Read the model definition and answer for the solid it produces. Units are mm, in the model's axes. A direction names the side the tool comes from. Give positions to 0.01 mm unless a question says otherwise; leave off trailing zeros. Loops run counter-clockwise (first coordinate to the right, second up) from the corner with the lowest first, then second, coordinate; pieces in that order, holes last. Notation, with made-up numbers: (-17, -31) - (39, -31) arc R18 cw to (39, -14) - close; hole circle Ø11 at (48.25, 23). An arc over 180 degrees is marked (long way). Write each question's results on one line, items separated by ' | '. Start each with the question number.
Q1. Find the intervals of material crossed by line 1 (X direction, y = 0, z = -17); line 2 (X direction, y = -11, z = -17); line 3 (Y direction, x = -15.5, z = 18), in increasing order. Write a range as from..to.
Q2. For faces 4 (the flat face through (-11.737, -10.552, -0.338)), 5 (the flat face through (0.838, 16, 0)), 6 (the flat face through (-0.838, -16, 0)), 7 (the flat face through (11.737, 10.552, -0.338)), determine the directions among +Z, -Z, +X, -X, +Y, -Y from which every point of the face is accessible in a straight line to the end or side of a thin tool.
Q3. The part is cut by section D-D, the plane y = -17. Write down the section's boundary in (x, z).
Q4. Given pin 1 (3 mm diameter, centred on x = -13, y = 7, fed in from +Z); pin 2 (12 mm diameter, centred on y = 3.5, z = -5.5, fed in from -X); pin 3 (5.5 mm diameter, centred on x = 16.5, z = 0, fed in from +Y); pin 4 (4 mm diameter, centred on x = -11.5, z = -8, fed in from -Y), each flat-ended and moving along its own axis, determine where each tip first touches the part or whether it passes through.
Q5. The part is cut by section A-A, the plane y = -9. Write down the section's boundary in (x, z).
Q6. The part is cut by section C-C, the plane y = 3. Write down the section's boundary in (x, z), plus the area to 3 significant figures.
Q7. Determine the mould class of faces 1 (the flat face through (-0.838, 16, 0)), 2 (the flat face through (-16, -0.838, 0)), 3 (the flat face through (0, -21.555, 0)) for opening direction Y: +Y half, -Y half, draft (parallel to the pull), parting line (faces both ways), or undercut.
Q8. The part is cut by section B-B, the plane x = 5. Write down the section's boundary in (y, z), plus the area to 3 significant figures.
Autodesk Inventor part; units mm, degrees
ref_plane "YZ Plane" through (0, 0, 0) normal (1, 0, 0) x (0, 1, 0)
ref_plane "XZ Plane" through (0, 0, 0) normal (0, 1, 0) x (-1, 0, 0)
ref_plane "XY Plane" through (0, 0, 0) normal (0, 0, 1) x (1, 0, 0)
sketch "Sketch1" plane through (0, 0, 0) normal (0, 0, 1) x (1, 0, 0)
  circle A0 centre (0, 0) radius 10.16
  circle A1 centre (0, 0) radius 8.5725
  line L0 (0.8382, 10.1254) -> (0.8382, 21.5554)
  line L1 (0.8382, 21.5554) -> (-0.8382, 21.5554)
  line L2 (-0.8382, 21.5554) -> (-0.8382, 10.1254)
  line L3 (-15.8346, 14.6492) -> (-7.7524, 6.567)
  line L4 (-14.6492, 15.8346) -> (-15.8346, 14.6492)
  line L5 (-6.567, 7.7524) -> (-14.6492, 15.8346)
  line L6 (-21.5554, -0.8382) -> (-10.1254, -0.8382)
  line L7 (-21.5554, 0.8382) -> (-21.5554, -0.8382)
  line L8 (-10.1254, 0.8382) -> (-21.5554, 0.8382)
  line L9 (-14.6492, -15.8346) -> (-6.567, -7.7524)
  line L10 (-15.8346, -14.6492) -> (-14.6492, -15.8346)
  line L11 (-7.7524, -6.567) -> (-15.8346, -14.6492)
  line L12 (0.8382, -21.5554) -> (0.8382, -10.1254)
  line L13 (-0.8382, -21.5554) -> (0.8382, -21.5554)
  line L14 (-0.8382, -10.1254) -> (-0.8382, -21.5554)
  line L15 (15.8346, -14.6492) -> (7.7524, -6.567)
  line L16 (14.6492, -15.8346) -> (15.8346, -14.6492)
  line L17 (6.567, -7.7524) -> (14.6492, -15.8346)
  line L18 (21.5554, 0.8382) -> (10.1254, 0.8382)
  line L19 (21.5554, -0.8382) -> (21.5554, 0.8382)
  line L20 (10.1254, -0.8382) -> (21.5554, -0.8382)
  line L21 (14.6492, 15.8346) -> (6.567, 7.7524)
  line L22 (15.8346, 14.6492) -> (14.6492, 15.8346)
  line L23 (7.7524, 6.567) -> (15.8346, 14.6492)
  line L24 (-7.479, 0) -> (-3.7395, 6.477)
  line L25 (-3.7395, 6.477) -> (3.7395, 6.477)
  line L26 (3.7395, 6.477) -> (7.479, 0)
  line L27 (7.479, 0) -> (3.7395, -6.477)
  line L28 (3.7395, -6.477) -> (-3.7395, -6.477)
  line L29 (-3.7395, -6.477) -> (-7.479, 0)
  point P0 (0, 21.5554)
  point P1 (-15.2419, 15.2419)
  point P2 (-21.5554, 0)
  point P3 (-15.2419, -15.2419)
  point P4 (0, -21.5554)
  point P5 (15.2419, -15.2419)
  point P6 (21.5554, 0)
  point P7 (15.2419, 15.2419)
  point P8 (-10.1254, -0.8382)
  point P9 (-10.1254, 0.8382)
  point P10 (-6.567, -7.7524)
  point P11 (-7.7524, -6.567)
  point P12 (0.8382, -10.1254)
  point P13 (-0.8382, -10.1254)
  point P14 (7.7524, -6.567)
  point P15 (6.567, -7.7524)
  point P16 (10.1254, 0.8382)
  point P17 (10.1254, -0.8382)
  point P18 (6.567, 7.7524)
  point P19 (7.7524, 6.567)
  point P20 (-7.7524, 6.567)
  point P21 (-6.567, 7.7524)
  dimension "d0" = 20.32
  dimension "d1" = 1.5875
  dimension "d7" = 1.6764
  dimension "d11" = 360
  dimension "d13" = 11.43
  dimension "d17" = 12.954
extrude "Extrusion1" add sketch "Sketch1" along normal mid plane 48.26 contours A0 | A0 L18 L19 L20 | A0 L21 L22 L23 | L15 L16 L17 A0 | A0 L2 L1 L0 | L12 L13 L14 A0 | A0 L3 L4 L5 | L9 L10 L11 A0 | A0 L6 L7 L8 | A1
properties part number "Spiral"
Check sheet entries:
1) line 1: x = -21.56..-7.48, 7.48..21.56 | line 2: x = -12.19..-9.81, -0.84..0.84, 9.81..12.19 | line 3: y = -14.98..-14.31, -0.84..0.84, 14.31..14.98
2) face 4: +Z, -Z, -X | face 5: +Z, -Z, +Y | face 6: +Z, -Z, -Y | face 7: +Z, -Z, +X
3) outline: (-0.84, -24.13) - (0.84, -24.13) - (0.84, 24.13) - (-0.84, 24.13) - close
4) pin 1: passes through | pin 2: stops at x = -21.56 | pin 3: stops at y = 15.83 | pin 4: stops at y = -14.69
5) outline: (-10.19, -24.13) - (-7.81, -24.13) - (-7.81, 24.13) - (-10.19, 24.13) - close; (-4.71, -24.13) - (4.71, -24.13) - (4.71, 24.13) - (-4.71, 24.13) - close; (7.81, -24.13) - (10.19, -24.13) - (10.19, 24.13) - (7.81, 24.13) - close
6) outline: (-9.71, -24.13) - (-5.75, -24.13) - (-5.75, 24.13) - (-9.71, 24.13) - close; (5.75, -24.13) - (9.71, -24.13) - (9.71, 24.13) - (5.75, 24.13) - close | area: 382 mm^2
7) face 1: draft | face 2: undercut | face 3: -Y half
8) outline: (-8.84, -24.13) - (-4.29, -24.13) - (-4.29, 24.13) - (-8.84, 24.13) - close; (4.29, -24.13) - (8.84, -24.13) - (8.84, 24.13) - (4.29, 24.13) - close | area: 439 mm^2
